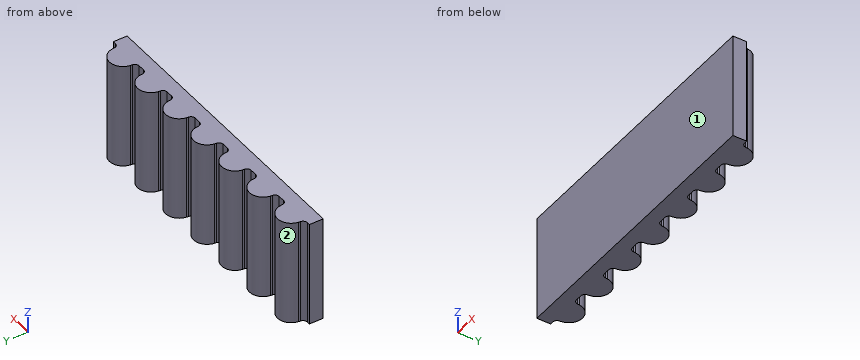
```python
from build123d import *

# Parameters (mm, degrees)
BOSS_EXTRUDE1_DEPTH = 20


with BuildPart() as part:
    # Sketch1 → Boss-Extrude1 (new body)
    with BuildSketch(Plane(origin=(0, 0, -10), x_dir=(-1, 0, 0), z_dir=(0, 0, -1))):
        with BuildLine():
            Line((0, 2.62), (-0.608434486, 2.62))
            ThreePointArc((-0.608434486, 2.62), (-1.142191341, 2.824094286), (-1.403606386, 3.33224095))
            Line((-1.403606386, 3.33224095), (-1.445510274, 3.711925947))
            ThreePointArc((-1.445510274, 3.711925947), (-4, 6), (-6.554489726, 3.711925947))
            Line((-6.554489726, 3.711925947), (-6.596393614, 3.33224095))
            ThreePointArc((-6.596393614, 3.33224095), (-6.857808659, 2.824094286), (-7.391565514, 2.62))
            Line((-7.391565514, 2.62), (-8.608434486, 2.62))
            ThreePointArc((-8.608434486, 2.62), (-9.142191341, 2.824094286), (-9.403606386, 3.33224095))
            Line((-9.403606386, 3.33224095), (-9.445510274, 3.711925947))
            ThreePointArc((-9.445510274, 3.711925947), (-12, 6), (-14.554489726, 3.711925947))
            Line((-14.554489726, 3.711925947), (-14.596393614, 3.33224095))
            ThreePointArc((-14.596393614, 3.33224095), (-14.857808659, 2.824094286), (-15.391565514, 2.62))
            Line((-15.391565514, 2.62), (-16.608434486, 2.62))
            ThreePointArc((-16.608434486, 2.62), (-17.142191341, 2.824094286), (-17.403606386, 3.33224095))
            Line((-17.403606386, 3.33224095), (-17.445510274, 3.711925947))
            ThreePointArc((-17.445510274, 3.711925947), (-20, 6), (-22.554489726, 3.711925947))
            Line((-22.554489726, 3.711925947), (-22.596393614, 3.33224095))
            ThreePointArc((-22.596393614, 3.33224095), (-22.857808659, 2.824094286), (-23.391565514, 2.62))
            Line((-23.391565514, 2.62), (-24.608434486, 2.62))
            ThreePointArc((-24.608434486, 2.62), (-25.142191341, 2.824094286), (-25.403606386, 3.33224095))
            Line((-25.403606386, 3.33224095), (-25.445510274, 3.711925947))
            ThreePointArc((-25.445510274, 3.711925947), (-28, 6), (-30.554489726, 3.711925947))
            Line((-30.554489726, 3.711925947), (-30.596393614, 3.33224095))
            ThreePointArc((-30.596393614, 3.33224095), (-30.857808659, 2.824094286), (-31.391565514, 2.62))
            Line((-31.391565514, 2.62), (-32.608434486, 2.62))
            ThreePointArc((-32.608434486, 2.62), (-33.142191341, 2.824094286), (-33.403606386, 3.33224095))
            Line((-33.403606386, 3.33224095), (-33.445510274, 3.711925947))
            ThreePointArc((-33.445510274, 3.711925947), (-36, 6), (-38.554489726, 3.711925947))
            Line((-38.554489726, 3.711925947), (-38.596393614, 3.33224095))
            ThreePointArc((-38.596393614, 3.33224095), (-38.857808659, 2.824094286), (-39.391565514, 2.62))
            Line((-39.391565514, 2.62), (-40.608434486, 2.62))
            ThreePointArc((-40.608434486, 2.62), (-41.142191341, 2.824094286), (-41.403606386, 3.33224095))
            Line((-41.403606386, 3.33224095), (-41.445510274, 3.711925947))
            ThreePointArc((-41.445510274, 3.711925947), (-44, 6), (-46.554489726, 3.711925947))
            Line((-46.554489726, 3.711925947), (-46.596393614, 3.33224095))
            ThreePointArc((-46.596393614, 3.33224095), (-46.857808659, 2.824094286), (-47.391565514, 2.62))
            Line((-47.391565514, 2.62), (-48.608434486, 2.62))
            ThreePointArc((-48.608434486, 2.62), (-49.142191341, 2.824094286), (-49.403606386, 3.33224095))
            Line((-49.403606386, 3.33224095), (-49.445510274, 3.711925947))
            ThreePointArc((-49.445510274, 3.711925947), (-52, 6), (-54.554489726, 3.711925947))
            Line((-54.554489726, 3.711925947), (-54.596393614, 3.33224095))
            ThreePointArc((-54.596393614, 3.33224095), (-54.857808659, 2.824094286), (-55.391565514, 2.62))
            Line((-55.391565514, 2.62), (-56, 2.62))
            Line((-56, 2.62), (-56, 0))
            Line((-56, 0), (0, 0))
            Line((0, 0), (0, 2.62))
        make_face()
    extrude(amount=-BOSS_EXTRUDE1_DEPTH)


solid = part.part
```
Model file for the job. Use its own axes, mm. Face numbers are marked on the shaded views. Coordinates: 2 decimals unless noted, no trailing zeros. Loops run counter-clockwise (first coordinate to the right, second up) from the corner with the lowest first, then second, coordinate; pieces in that order, holes last. Notation, with made-up numbers: (39.5, 30.5) - (66.5, 30.5) arc R14 cw to (66.5, 53.5) - close; hole circle Ø11 at (56, 82). An arc over 180 degrees is marked (long way). Write item = value, one per line. Start each with the question number.
Item 1: Pull direction X, two halves, no side cores. Call the marked faces 1 and 2: +X half, -X half, draft (parallel to the pull), parting line (faces both ways), or undercut.
Item 2: Wall check: probe 1 along Y at (x, z) = (32, -8.75); probe 2 along Y at (x, z) = (35.5, 4.25). Give the ranges that are in metal, low to high. Write a range as [from, to].
Item 3: Drop a flat-ended pin along its axis: pin 1 Ø1.3 at (x, z) = (32, -3) entering from +Y. Give the stop position or say it passes through.
Item 4: Saw through at A-A, the plane y = 4.2. List the corners of the cut face in (x, z), then the cut area to 3 significant figures.
Item 5: Saw through at B-B, the plane x = 11. List the corners of the cut face in (y, z), then the cut area to 3 significant figures.
Answers:
q1.face_1 = draft
q1.face_2 = undercut
q2.probe_1 = [0, 2.62]
q2.probe_2 = [0, 5.95]
q3.pin_1 = 2.62
q4.outline = (1.55, -10) - (6.45, -10) - (6.45, 10) - (1.55, 10) - close; (9.55, -10) - (14.45, -10) - (14.45, 10) - (9.55, 10) - close; (17.55, -10) - (22.45, -10) - (22.45, 10) - (17.55, 10) - close; (25.55, -10) - (30.45, -10) - (30.45, 10) - (25.55, 10) - close; (33.55, -10) - (38.45, -10) - (38.45, 10) - (33.55, 10) - close; (41.55, -10) - (46.45, -10) - (46.45, 10) - (41.55, 10) - close; (49.55, -10) - (54.45, -10) - (54.45, 10) - (49.55, 10) - close
q4.area = 687 mm2
q5.outline = (0, -10) - (5.8, -10) - (5.8, 10) - (0, 10) - close
q5.area = 116 mm2
